from build123d import *

# Parameters (mm, degrees)
SKETCH1_R           = 25.5
SKETCH1_R_2         = 18
SKETCH1_R_3         = 3.7
BOSS_EXTRUDE1_DEPTH = 1
SKETCH1_3_R         = 18
SKETCH1_3_R_2       = 3.7
BOSS_EXTRUDE2_DEPTH = 1.8
HOLE1_D             = 3.2
HOLE1_DEPTH         = 7.857098765
HOLE1_CSINK_D       = 6.2
HOLE1_CSINK_ANGLE   = 86


with BuildPart() as part:
    # Sketch1 → Boss-Extrude1 (new body)
    # profile 1 of 2: a face of its own
    with BuildSketch(Plane(origin=(0, 0, 0), x_dir=(1, 0, 0), z_dir=(0, 1, 0))):
        with Locations(Location((0, 0, 0), (0, 0, 270))):
            Circle(SKETCH1_R)
        Circle(SKETCH1_R_2, mode=Mode.SUBTRACT)
    # profile 2 of 2: a face of its own
    with BuildSketch(Plane(origin=(0, 0, 0), x_dir=(1, 0, 0), z_dir=(0, 1, 0))):
        Circle(SKETCH1_R_2)
        with Locations(Location((0, 0, 0), (0, 0, 270))):
            Circle(SKETCH1_R_3, mode=Mode.SUBTRACT)
    extrude(amount=BOSS_EXTRUDE1_DEPTH)

    # Sketch1_3 → Boss-Extrude2 (add)
    with BuildSketch(Plane(origin=(0, 0, 0), x_dir=(1, 0, 0), z_dir=(0, 1, 0))):
        with Locations(Location((0, 0, 0), (0, 0, 270))):
            Circle(SKETCH1_3_R)
        with Locations(Location((0, 0, 0), (0, 0, 270))):
            Circle(SKETCH1_3_R_2, mode=Mode.SUBTRACT)
    extrude(amount=BOSS_EXTRUDE2_DEPTH)

    # Hole1
    with Locations(Plane(origin=(7.317914662, 1.8, -4.225), x_dir=(0, 0, 1), z_dir=(0, 1, 0))):
        with Locations((0, 0), (0, -14.635829324), (12.675, -7.317914662)):
            CounterSinkHole(HOLE1_D / 2, HOLE1_CSINK_D / 2, depth=HOLE1_DEPTH, counter_sink_angle=HOLE1_CSINK_ANGLE)


solid = part.part
The listing builds one solid part. Answer for the finished solid, in the listing's coordinates (mm). A direction names the side the tool comes from. Round coordinates to 2 decimals unless told otherwise and drop trailing zeros. Loops run counter-clockwise (first coordinate to the right, second up) from the corner with the lowest first, then second, coordinate; pieces in that order, holes last. Notation, with made-up numbers: M 79,51.5 L 101,51.5 A20 ccw 101,89.5 Z; hole C 50,7 d6. An arc over 180 degrees is marked long. Write each question's results on one line, items separated by ' | '. Start each with the question number.
1) Find section C-C on z = 8.45. Write down the section's boundary in (x, y), plus the area to 3 significant figures.
2) Which of the six approach directions +Z, -Z, +X, -X, +Y, -Y give full straight-line access (tool end or side, diameter ignored) to faces 4 (the cylindrical face through (-24.9, 0.5, -5.5)), 5 (the flat face through (-17.4, 1, 5.3))?
3) Find section D-D on x = -14. Write down the section's boundary in (y, z), plus the area to 3 significant figures.
4) Determine the mould class of faces 1 (the cylindrical face through (-3.612, 0.887, -0.802)), 2 (the flat face through (-4, 1.8, 0)), 3 (the cylindrical face through (5.407, 1.394, 17.169)) for opening direction X: pulls with the +X half, pulls with the -X half, needs draft (parallel to the pull), parting line crosses it, or undercut.
5) Find section B-B on y = 1.3. Write down the section's boundary in (x, z) (3 decimals).
6) Find section A-A on z = 0. Write down the section's boundary in (x, y), plus the area to 3 significant figures.
7) Each of these flat-tipped pins is pushed along its axis until it touches: pin 1 (5 mm diameter, centred on x = 0, z = 8.45, fed in from +Y); pin 2 (8 mm diameter, centred on x = -12.5, z = -19, fed in from +Y). Where does it stop, or does it pass through?
8) Straight lines are drawn through the part: probe 1 along X at (y, z) = (0.6, 0); probe 2 along X at (y, z) = (0.65, -6); probe 3 along Y at (x, z) = (-17, -6.5). For each, find the intervals that lie inside material, in ascending order.
Final values:
1) outline: M -24.06,0 L -1.6,0 L -1.6,0.19 L -3.1,1.8 L -15.89,1.8 L -15.89,1 L -24.06,1 Z; M 1.6,0 L 24.06,0 L 24.06,1 L 15.89,1 L 15.89,1.8 L 3.1,1.8 L 1.6,0.19 Z | area: 65.4 mm²
2) face 4: +Y, -Y | face 5: +Y
3) outline: M 0,-21.31 L 1,-21.31 L 1,-11.31 L 1.8,-11.31 L 1.8,11.31 L 1,11.31 L 1,21.31 L 0,21.31 Z | area: 60.7 mm²
4) face 1: undercut | face 2: needs draft | face 3: parting line crosses it
5) outline: C 0,0 d36; hole C -7.318,-4.225 d5.267; hole C 0,0 d7.4; hole C 0,8.45 d5.267; hole C 7.318,-4.225 d5.267
6) outline: M -25.5,0 L -3.7,0 L -3.7,1.8 L -18,1.8 L -18,1 L -25.5,1 Z; M 3.7,0 L 25.5,0 L 25.5,1 L 18,1 L 18,1.8 L 3.7,1.8 Z | area: 66.5 mm²
7) pin 1: y = 1.16 | pin 2: y = 1
8) probe 1: -25.5 to -3.7, 3.7 to 25.5 | probe 2: -24.78 to -8.3, -6.34 to 6.34, 8.3 to 24.78 | probe 3: 0 to 1
